from build123d import *

# Parameters (mm, degrees)
SKETCH1_W           = 15
SKETCH1_H           = 15
BOSS_EXTRUDE1_DEPTH = 3
SKETCH2_R           = 6
SKETCH2_R_2         = 2.5
CUT_EXTRUDE1_DEPTH  = 2
SKETCH3_R           = 1.25
CUT_EXTRUDE2_DEPTH  = 2


with BuildPart() as part:
    # Sketch1 → Boss-Extrude1 (new body)
    with BuildSketch(Plane(origin=(0, 0, 0), x_dir=(1, 0, 0), z_dir=(0, 1, 0))):
        Rectangle(SKETCH1_W, SKETCH1_H)
    extrude(amount=BOSS_EXTRUDE1_DEPTH)

    # Sketch2 → Cut-Extrude1 (cut)
    with BuildSketch(Plane.XZ):
        Circle(SKETCH2_R)
        Circle(SKETCH2_R_2, mode=Mode.SUBTRACT)
    extrude(amount=-CUT_EXTRUDE1_DEPTH, mode=Mode.SUBTRACT)

    # Sketch3 → Cut-Extrude2 (cut)
    with BuildSketch(Plane.XZ):
        with Locations((5.5, 5.5)):
            Circle(SKETCH3_R)
        with Locations((-5.5, 5.5)):
            Circle(SKETCH3_R)
        with Locations((-5.5, -5.5)):
            Circle(SKETCH3_R)
        with Locations((5.5, -5.5)):
            Circle(SKETCH3_R)
    extrude(amount=-CUT_EXTRUDE2_DEPTH, mode=Mode.SUBTRACT)


solid = part.part
Design review of the part built by this model. Coordinates are the model's own, in mm. A direction names the side the tool comes from. Round coordinates to 2 decimals unless told otherwise and drop trailing zeros. Write each loop counter-clockwise with the first axis right and the second up, starting at its lowest first coordinate (ties: lowest second). Pieces come first, ordered by that corner, then holes. Notation, with made-up numbers: (-7.5, 74.25) -> (48.5, 74.25) arc R24 cw to (48.5, 111.25) -> close; hole circle Ø5 at (85.5, 80.5). An arc over 180 degrees is marked (long way). One line per question, with ' | ' between items.
(1) Machinability: for faces 1 (the flat face through (0, 3, 0)), 2 (the flat face through (5, 2, -5)), which of the approach directions +Z, -Z, +X, -X, +Y, -Y give a long, thin tool a straight path to every point of the face, cutting with its end or side? Answer none if there is none.
Result sheet:
face 1: +Z, -Z, +X, -X, +Y | face 2: -Y
(2) Insertion check: P1, Ø3, axis at x = -5, z = -5, coming from the -Y side; P2, Ø1.2, axis at x = -5.5, z = 6, coming from the -Y side. Each pin has a flat end and moves straight along its axis. Give the tip position at first contact, or say it passes through.
Result sheet:
P1: y = 0 | P2: y = 2
(3) Take a section at D-D, the plane x = -5. State the section outline as (y, z) points, and give its area (3 significant figures).
Result sheet:
outline: (0, -7.5) -> (3, -7.5) -> (3, 7.5) -> (0, 7.5) -> (0, 6.65) -> (2, 6.65) -> (2, 4.35) -> (0, 4.35) -> (0, 3.32) -> (2, 3.32) -> (2, -3.32) -> (0, -3.32) -> (0, -4.35) -> (2, -4.35) -> (2, -6.65) -> (0, -6.65) -> close | area: 22.6 mm2
(4) Take a section at B-B, the plane x = 6.5. State the section outline as (y, z) points, and give its area (3 significant figures).
Result sheet:
outline: (0, -7.5) -> (3, -7.5) -> (3, 7.5) -> (0, 7.5) -> (0, 6.25) -> (2, 6.25) -> (2, 4.75) -> (0, 4.75) -> (0, -4.75) -> (2, -4.75) -> (2, -6.25) -> (0, -6.25) -> close | area: 39.0 mm2
(5) Take a section at A-A, the plane y = 1.8. State the section outline as (x, z) points.
Result sheet:
outline: (-7.5, -7.5) -> (7.5, -7.5) -> (7.5, 7.5) -> (-7.5, 7.5) -> close; circle Ø5 at (0, 0); hole circle Ø2.5 at (-5.5, -5.5); hole circle Ø2.5 at (-5.5, 5.5); hole circle Ø12 at (0, 0); hole circle Ø2.5 at (5.5, -5.5); hole circle Ø2.5 at (5.5, 5.5)
(6) Take a section at C-C, the plane z = 0. State the section outline as (x, y) points, and give its area (3 significant figures).
Result sheet:
outline: (-7.5, 0) -> (-6, 0) -> (-6, 2) -> (-2.5, 2) -> (-2.5, 0) -> (2.5, 0) -> (2.5, 2) -> (6, 2) -> (6, 0) -> (7.5, 0) -> (7.5, 3) -> (-7.5, 3) -> close | area: 31.0 mm2
(7) Draft analysis for pull direction X (two halves, no side actions). For faces 3 (the flat face through (-3.44, 0, -5.1)), 4 (the cylindrical face through (-5.77, 0.99, 4.28)), 5 (the flat face through (7.5, 1, 0)), state which applies: released by +X, released by -X, zero draft, split by the parting line, or undercut.
Result sheet:
face 3: zero draft | face 4: undercut | face 5: released by +X
(8) Wall thickness on line 1 (Z direction, x = 0, y = 0.65); line 2 (X direction, y = 0.95, z = -4.5); line 3 (Z direction, x = 5, y = 1.45): over which ranges is each line inside the solid? List them lowest first. Write a range as [from, to].
Result sheet:
line 1: [-7.5, -6], [-2.5, 2.5], [6, 7.5] | line 2: [-7.5, -6.25], [-4.75, -3.97], [3.97, 4.75], [6.25, 7.5] | line 3: [-7.5, -6.65], [-4.35, -3.32], [3.32, 4.35], [6.65, 7.5]
